Answer from the drawing. Dimensions are ordinates in mm from the lowest x, y and z of the part. Round coordinates to 2 decimals unless told otherwise and drop trailing zeros. Write each loop counter-clockwise with the first axis right and the second up, starting at its lowest first coordinate (ties: lowest second). Pieces come first, ordered by that corner, then holes. Notation, with made-up numbers: (-7, 66) - (12, 66) arc R25 cw to (12, 82) - close; hole circle Ø7 at (20.25, 44). An arc over 180 degrees is marked (long way). Return JSON: item names as keys, results as strings. Group by question number.
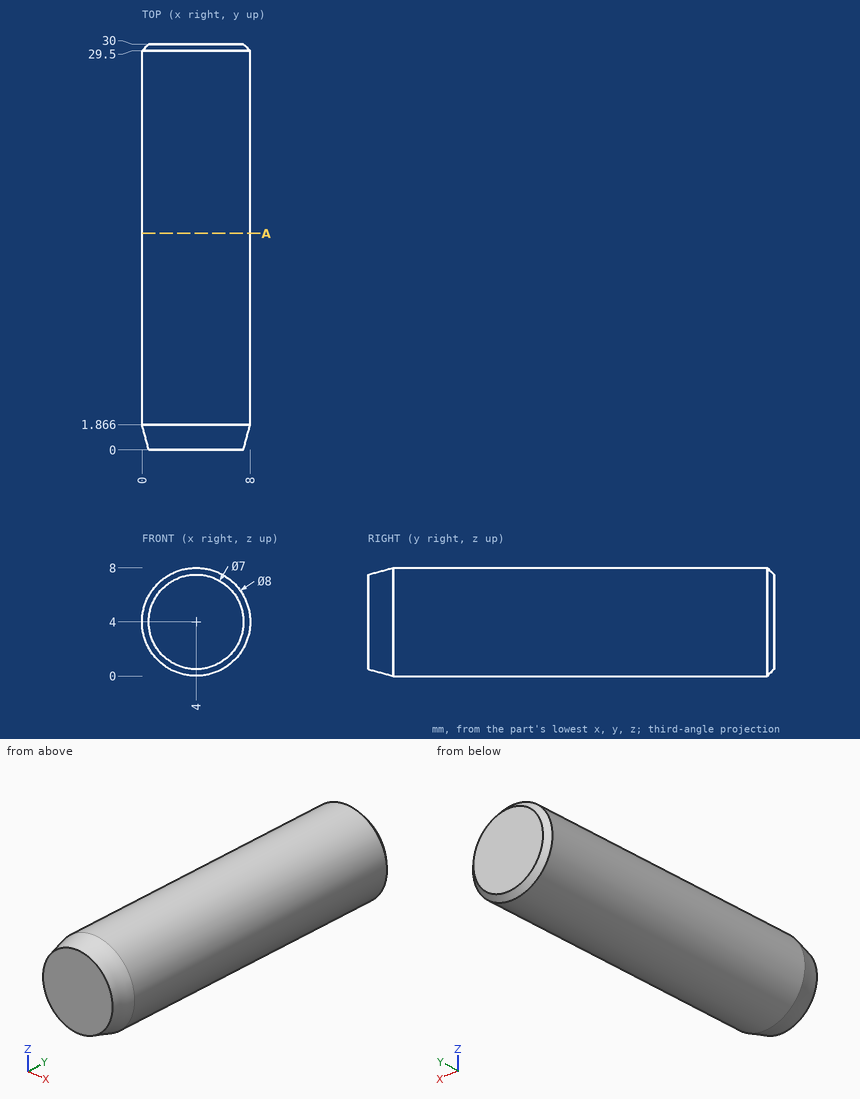
(1) Flat-ended cylindrical pins translate along their axes: pin 1 (2 mm diameter, centred on x = 2.5, y = 13, fed in from -Z); pin 2 (1.5 mm diameter, centred on x = 6.5, y = 8, fed in from +Z). Find the tip coordinate at first contact, or state that the pin passes through.
(2) Consider line 1 (Z direction, x = 6, y = 20.5); line 2 (Z direction, x = 2.25, y = 16); line 3 (X direction, y = 7.5, z = 2.75). Determine where each line is inside the solid, lowest interval first.
(3) Find section A-A (y = 16). Write down the section's boundary in (x, z), plus the area to 3 significant figures.
Check sheet entries:
{
 "1": {"pin 1": "stops at z = 0.03", "pin 2": "stops at z = 7.6"},
 "2": {"line 1": "z = 0.54 to 7.46", "line 2": "z = 0.4 to 7.6", "line 3": "x = 0.2 to 7.8"},
 "3": {"outline": "circle Ø8 at (4, 4)", "area": "50.3 mm^2"}
}
